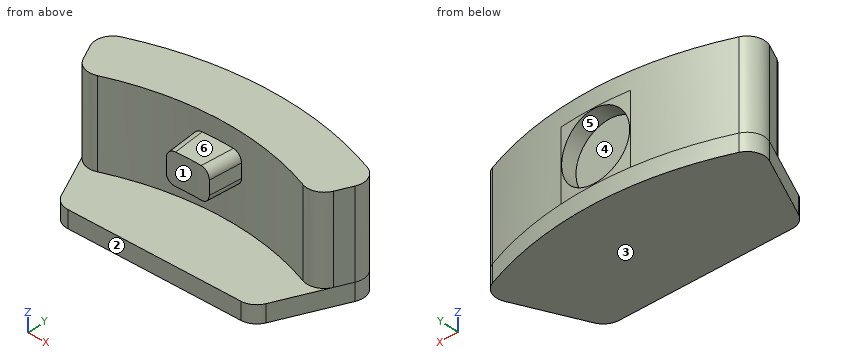
from build123d import *

# Parameters (mm, degrees)
EXTRUDE_1_DEPTH      = 5
SKETCH_2_W           = 1.8
SKETCH_2_H           = 3.7
REVOLVE_1_ANGLE      = 5
FILLET_1_R           = 0.5
FILLET_2_R           = 1
FILLET_3_R           = 1
SKETCH_4_W           = 4
SKETCH_4_H           = 2
CUT_EXTRUDE_1_DEPTH  = 4
EXTRUDE_5_REACH      = 11.968
EXTRUDE_5_END_RADIUS = 19
SKETCH_5_W           = 4
SKETCH_5_H           = 4
SKETCH_5_R           = 1.95
EXTRUDE_6_DEPTH      = 1
FILLET_5_R           = 1


with BuildPart() as part:
    # 草图1 → 凸台-拉伸1 (new body)
    with BuildSketch(Plane.XY):
        with BuildLine():
            Line((-8.029746973, 17.219847954), (-6.761892188, 14.500924593))
            ThreePointArc((-6.761892188, 14.500924593), (0, 16), (6.761892188, 14.500924593))
            Line((6.761892188, 14.500924593), (8.029746973, 17.219847954))
            ThreePointArc((8.029746973, 17.219847954), (0, 19), (-8.029746973, 17.219847954))
        make_face()
    extrude(amount=EXTRUDE_1_DEPTH)

    # 草图2 → 旋转1 (revolve)
    with BuildSketch(Plane(origin=(0, 0, 0), x_dir=(0, 0, -1), z_dir=(1, 0, 0))):
        with Locations((-3, 16)):
            Rectangle(SKETCH_2_W, SKETCH_2_H)
    revolve_1 = revolve(axis=Axis((0, 0, 5), (0, 0, -1)), revolution_arc=REVOLVE_1_ANGLE)

    # 镜向1: 旋转1 across plane
    add(revolve_1.mirror(Plane(origin=(0, 0, 0), x_dir=(0, 0, 1), z_dir=(1, 0, 0))))

    # 圆角1
    fillet_1_edges = [part.edges().sort_by_distance(p)[0] for p in [
        (1.313872822, 15.017635074, 3.9),
        (1.313872822, 15.017635074, 2.1),
        (-1.313872822, 15.017635074, 2.1),
        (-1.313872822, 15.017635074, 3.9),
    ]]
    fillet(fillet_1_edges, radius=FILLET_1_R)

    # 圆角2
    fillet_2_edges = [part.edges().sort_by_distance(p)[0] for p in [
        (-6.761892188, 14.500924593, 2.5),
        (6.761892188, 14.500924593, 2.5),
    ]]
    fillet(fillet_2_edges, radius=FILLET_2_R)

    # 圆角3
    fillet_3_edges = [part.edges().sort_by_distance(p)[0] for p in [
        (-8.029746973, 17.219847954, 2.5),
        (8.029746973, 17.219847954, 2.5),
    ]]
    fillet(fillet_3_edges, radius=FILLET_3_R)

    # 草图4 → 切除-拉伸1 (cut)
    with BuildSketch(Plane(origin=(0, 0, 0), x_dir=(-1, 0, 0), z_dir=(0, 0, -1))):
        with Locations((0, 19)):
            Rectangle(SKETCH_4_W, SKETCH_4_H)
    extrude(amount=-CUT_EXTRUDE_1_DEPTH, mode=Mode.SUBTRACT)

    # 凸台-拉伸5: up to this cylinder (the profile starts inside it)
    extrude_5_end = Plane(origin=(0, 0, 3.994343), z_dir=(0, 0, -1)) * Cylinder(EXTRUDE_5_END_RADIUS, 62.936, mode=Mode.PRIVATE)
    # 草图5 → 凸台-拉伸5 (add, up to the surface)
    with BuildSketch(Plane(origin=(0, 18, 0), x_dir=(1, 0, 0), z_dir=(0, 1, 0)), mode=Mode.PRIVATE) as extrude_5_sk1:
        with Locations((0, -2)):
            Rectangle(SKETCH_5_W, SKETCH_5_H)
        with Locations(Location((0, -2, 0), (0, 0, 90))):
            Circle(SKETCH_5_R, mode=Mode.SUBTRACT)
    extrude_5_tool1 = extrude(extrude_5_sk1.sketch, amount=EXTRUDE_5_REACH, mode=Mode.PRIVATE) & extrude_5_end
    add(extrude_5_tool1.solids().sort_by_distance((0, 18, 3.994343))[0])

    # 草图6 → 凸台-拉伸6 (add)
    with BuildSketch(Plane(origin=(0, 0, 0), x_dir=(-1, 0, 0), z_dir=(0, 0, -1))):
        with BuildLine():
            Line((-7.595380243, 16.288345495), (-5.595691898, 12))
            Line((-5.595691898, 12), (5.595691898, 12))
            Line((5.595691898, 12), (7.595380243, 16.288345495))
            ThreePointArc((7.595380243, 16.288345495), (7.618897961, 17.078964477), (7.060687592, 17.639350632))
            ThreePointArc((7.060687592, 17.639350632), (0, 19), (-7.060687592, 17.639350632))
            ThreePointArc((-7.060687592, 17.639350632), (-7.618897961, 17.078964477), (-7.595380243, 16.288345495))
        make_face()
    extrude(amount=EXTRUDE_6_DEPTH)

    # 圆角5
    fillet_5_edges = [part.edges().sort_by_distance(p)[0] for p in [
        (5.595691898, 12, -0.5),
        (-5.595691898, 12, -0.5),
    ]]
    fillet(fillet_5_edges, radius=FILLET_5_R)


solid = part.part
Geometry check sheet. Reference: the model listing, model coordinates, mm. Face numbers are marked on the shaded views. A direction names the side the tool comes from. Give positions to 0.01 mm unless a question says otherwise; leave off trailing zeros. Loops run counter-clockwise (first coordinate to the right, second up) from the corner with the lowest first, then second, coordinate; pieces in that order, holes last. Notation, with made-up numbers: (0.5, -20) -> (50.5, -20) arc R10 ccw to (50.5, -16) -> close; hole circle Ø9 at (-14.5, -35). An arc over 180 degrees is marked (long way). Answer in a Markdown table with one row per item. Add a question column.
1) Cross-section at A-A on z = 4.25. Record the boundary of the cut face in (x, y), and give its area (3 significant figures).
2) Cross-section at D-D on z = -0.5. Record the boundary of the cut face in (x, y), and give its area (3 significant figures).
3) Draft check along Z on the marked faces 3, 4, 5 and 6. Enter one of: pulls with the +Z half, pulls with the -Z half, needs draft (parallel to the pull), parting line crosses it, or undercut.
4) Set-up check for the marked faces 1 and 2: record each of +Z, -Z, +X, -X, +Y, -Y from which the full face is reachable in a straight line by a thin tool's end or side.
5) Gauge pin test, flat ends, axial feed: P1, Ø1.2, axis at x = 3, y = 13.5, coming from the +Z side; P2, Ø3, axis at x = 0, z = 2, coming from the +Y side; P3, Ø1, axis at x = -5, z = 3.5, coming from the +Y side. Record the tip position at first contact, or that the pin passes through.
6) Cross-section at C-C on x = 0. Record the boundary of the cut face in (y, z), and give its area (3 significant figures).
7) Material ranges on probe 1 along Z at (x, y) = (4.5, 14.75); probe 2 along Y at (x, z) = (-3.25, 1); probe 3 along Y at (x, z) = (0, 4), recorded low to high. Write a range as from..to.
8) Cross-section at B-B on y = 18.75. Record the boundary of the cut face in (x, z), and give its area (3 significant figures).
Outcome:
| question | item | result |
|---|---|---|
| 1 | outline | (-7.6, 16.29) -> (-7.17, 15.38) arc R1 ccw to (-5.9, 14.87) arc R16 cw to (5.9, 14.87) arc R1 ccw to (7.17, 15.38) -> (7.6, 16.29) arc R1 ccw to (7.06, 17.64) arc R19 ccw to (-7.06, 17.64) arc R1 ccw to start |
| 1 | area | 45.0 mm^2 |
| 2 | outline | (-7.6, 16.29) -> (-5.86, 12.58) arc R1 ccw to (-4.96, 12) -> (4.96, 12) arc R1 ccw to (5.86, 12.58) -> (7.6, 16.29) arc R1 ccw to (7.06, 17.64) arc R19 ccw to (-7.06, 17.64) arc R1 ccw to start |
| 2 | area | 89.8 mm^2 |
| 3 | face 3 | pulls with the -Z half |
| 3 | face 4 | undercut |
| 3 | face 5 | undercut |
| 3 | face 6 | pulls with the +Z half |
| 4 | face 1 | +Z, -Y |
| 4 | face 2 | +Z, -Z, +X, -X, -Y |
| 5 | P1 | stops at z = 0 |
| 5 | P2 | stops at y = 18 |
| 5 | P3 | stops at y = 18.46 |
| 6 | outline | (12, -1) -> (19, -1) -> (19, 0.05) -> (18, 0.05) -> (18, 3.95) -> (19, 3.95) -> (19, 5) -> (16, 5) -> (16, 3.9) -> (14.15, 3.9) -> (14.15, 2.1) -> (16, 2.1) -> (16, 0) -> (12, 0) -> close |
| 6 | area | 21.4 mm^2 |
| 7 | probe 1 | z = -1..0 |
| 7 | probe 2 | y = 15.67..18.72 |
| 7 | probe 3 | y = 16..19 |
| 8 | outline | (-3.07, -1) -> (3.07, -1) -> (3.07, 5) -> (-3.07, 5) -> close; hole circle Ø3.9 at (0, 2) |
| 8 | area | 24.9 mm^2 |
